Autodesk Inventor part; units mm, degrees
ref_plane "YZ Plane" through (0, 0, 0) normal (1, 0, 0) x (0, 1, 0)
ref_plane "XZ Plane" through (0, 0, 0) normal (0, 1, 0) x (-1, 0, 0)
ref_plane "XY Plane" through (0, 0, 0) normal (0, 0, 1) x (1, 0, 0)
sketch "Sketch1" plane through (0, 0, 0) normal (0, 0, 1) x (1, 0, 0)
  circle A0 centre (0, 0) radius 2.6
  circle A1 centre (0, 0) radius 3.5
  dimension "d0" = 5.2
  dimension "d1" = 7
extrude "Extrusion1" add sketch "Sketch1" along normal blind 15
sketch "Sketch2" plane through (0, 0, 15) normal (0, 0, 1) x (1, 0, 0)
  circle A0 centre (0, 0) radius 2.6
  circle A1 centre (0, 0) radius 3.75
  line L0 (-6, 0.85) -> (6, 0.85)
  line L1 (6, 0.85) -> (6, -0.85)
  line L2 (6, -0.85) -> (-6, -0.85)
  line L3 (-6, -0.85) -> (-6, 0.85)
  line L4 (-6, 0.85) -> (6, -0.85) construction
  line L5 (6, 0.85) -> (-6, -0.85) construction
  point P0 (-3.6524, 0.85)
  point P1 (-3.6524, -0.85)
  point P2 (3.6524, -0.85)
  point P3 (3.6524, 0.85)
  dimension "d4" = 7.5
  dimension "d5" = 12
  dimension "d6" = 1.7
extrude "Extrusion2" add sketch "Sketch2" along normal blind 25 contours A0 L0 A1 L2 | A0 L0 A1 | L2 A1 A0 | A0 L2 A1 L0 | L0 L1 L2 A1 | A1 L2 L3 L0
sketch "Sketch3" plane through (0, 0, 0) normal (0, 0, -1) x (-1, 0, 0)
  point P0 (0, 0)
properties part number "final pin_3DPrint"
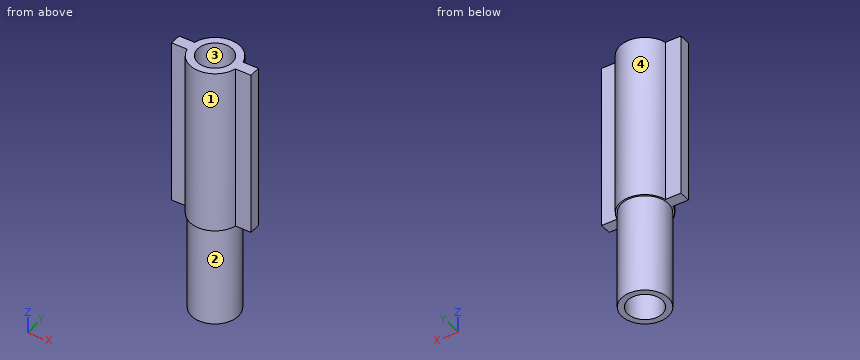
The listing builds one solid part. Answer for the finished solid, in the listing's coordinates (mm). Face numbers are marked on the shaded views. A direction names the side the tool comes from. Round coordinates to 2 decimals unless told otherwise and drop trailing zeros. Write each loop counter-clockwise with the first axis right and the second up, starting at its lowest first coordinate (ties: lowest second). Pieces come first, ordered by that corner, then holes. Notation, with made-up numbers: (-39.75, 68) -> (-1.75, 68) arc R21 ccw to (-1.75, 80) -> close; hole circle Ø2 at (47, 70.5). An arc over 180 degrees is marked (long way). Answer as a JSON object with one key per item and string values. Group by question number.
Q1. Which of the six approach directions +Z, -Z, +X, -X, +Y, -Y give full straight-line access (tool end or side, diameter ignored) to the marked faces 1 and 2?
Q2. Section C-C (x = 0) is taken. Write down the section's boundary in (y, z).
Q3. Section A-A (y = 0) is taken. Write down the section's boundary in (x, z), plus the area to 3 significant figures.
Q4. Straight lines are drawn through the part: line 1 along Y through (x, z) = (0, 10.5); line 2 along Y through (x, z) = (0, 23.5); line 3 along X through (y, z) = (2.25, 2). For each, find the intervals that lie inside material, in ascending order.
Q5. Each of these flat-tipped pins is pushed along its axis until it touches: pin 1 Ø2 at (y, z) = (-2, 22) entering from +X; pin 2 Ø1 at (x, z) = (2.5, 23) entering from -Y; pin 3 Ø2.5 at (x, z) = (-5, 21.5) entering from -Y. Where does it stop, or does it pass through?
Q6. Section D-D (x = 3) is taken. Write down the section's boundary in (y, z), plus the area to 3 significant figures.
Q7. Determine the mould class of the marked faces 3 and 4 for opening direction X: pulls with the +X half, pulls with the -X half, needs draft (parallel to the pull), parting line crosses it, or undercut.
Q8. Section B-B (z = 26.5) is taken. Write down the section's boundary in (x, y).
Check values:
{
 "1": {"face 1": "+Z, -Z, -Y", "face 2": "-Z"},
 "2": {"outline": "(-3.75, 15) -> (-3.5, 15) -> (-3.5, 0) -> (-2.6, 0) -> (-2.6, 40) -> (-3.75, 40) -> close; (2.6, 0) -> (3.5, 0) -> (3.5, 15) -> (3.75, 15) -> (3.75, 40) -> (2.6, 40) -> close"},
 "3": {"outline": "(-6, 15) -> (-3.5, 15) -> (-3.5, 0) -> (-2.6, 0) -> (-2.6, 40) -> (-6, 40) -> close; (2.6, 0) -> (3.5, 0) -> (3.5, 15) -> (6, 15) -> (6, 40) -> (2.6, 40) -> close", "area": "197 mm^2"},
 "4": {"line 1": "-3.5 to -2.6, 2.6 to 3.5", "line 2": "-3.75 to -2.6, 2.6 to 3.75", "line 3": "-2.68 to -1.3, 1.3 to 2.68"},
 "5": {"pin 1": "x = 3.61", "pin 2": "y = -3.17", "pin 3": "y = -0.85"},
 "6": {"outline": "(-2.25, 15) -> (-1.8, 15) -> (-1.8, 0) -> (1.8, 0) -> (1.8, 15) -> (2.25, 15) -> (2.25, 40) -> (-2.25, 40) -> close", "area": "167 mm^2"},
 "7": {"face 3": "undercut", "face 4": "parting line crosses it"},
 "8": {"outline": "(-6, -0.85) -> (-3.65, -0.85) arc R3.75 ccw to (3.65, -0.85) -> (6, -0.85) -> (6, 0.85) -> (3.65, 0.85) arc R3.75 ccw to (-3.65, 0.85) -> (-6, 0.85) -> close; hole circle Ø5.2 at (0, 0)"}
}
